Part model, mm, in its own coordinate system. Face numbers are marked on the shaded views. A direction names the side the tool comes from. Round coordinates to 2 decimals unless told otherwise and drop trailing zeros. Loops run counter-clockwise (first coordinate to the right, second up) from the corner with the lowest first, then second, coordinate; pieces in that order, holes last. Notation, with made-up numbers: (5, -26.5) - (27, -26.5) arc R23 ccw to (27, -1.5) - close; hole circle Ø1 at (30.25, -29). An arc over 180 degrees is marked (long way). Put each result on its own line as item: value.
from build123d import *

# Parameters (mm, degrees)
ESQUISSE1_R                  = 100
ESQUISSE1_R_2                = 4.25
ESQUISSE1_R_3                = 8
BOSS_EXTRU_1_DEPTH           = 40
ESQUISSE3_R                  = 5
ENL_V_MAT_EXTRU_2_DEPTH      = 41
ESQUISSE5_R                  = 15
ENL_V_MAT_EXTRU_3_DEPTH      = 30
ESQUISSE6_R                  = 33
ENL_V_MAT_EXTRU_4_DEPTH      = 5
ESQUISSE8_R                  = 17
ENL_V_MAT_EXTRU_5_DEPTH      = 20
R_P_TITION_CIRCULAIRE1_COUNT = 3


with BuildPart() as part:
    # Esquisse1 → Boss.-Extru.1 (new body)
    with BuildSketch(Plane(origin=(0, 0, 0), x_dir=(1, 0, 0), z_dir=(0, 1, 0))):
        with Locations(Location((0, 0, 0), (0, 0, 270))):  # turned: the seam where the file's is
            Circle(ESQUISSE1_R)
        with Locations(Location((-40.311740852, 7.648092634, 0), (0, 0, 270))):  # turned: the seam where the file's is
            Circle(ESQUISSE1_R_2, mode=Mode.SUBTRACT)
        with Locations(Location((-68.947262615, 13.080929779, 0), (0, 0, 270))):  # turned: the seam where the file's is
            Circle(ESQUISSE1_R_3, mode=Mode.SUBTRACT)
        with Locations(Location((45.802048801, 53.169616056, 0), (0, 0, 270))):  # turned: the seam where the file's is
            Circle(ESQUISSE1_R_3, mode=Mode.SUBTRACT)
        with Locations(Location((23.145213813, -66.250545836, 0), (0, 0, 270))):  # turned: the seam where the file's is
            Circle(ESQUISSE1_R_3, mode=Mode.SUBTRACT)
    extrude(amount=-BOSS_EXTRU_1_DEPTH)

    # Esquisse3 → Enlèv. mat.-Extru.2 (cut, through all)
    with BuildSketch(Plane(origin=(0, 0, 0), x_dir=(1, 0, 0), z_dir=(0, 1, 0))):
        with Locations(Location((0, 0, 0), (0, 0, 270))):  # turned: the seam where the file's is
            Circle(ESQUISSE3_R)
    extrude(amount=-ENL_V_MAT_EXTRU_2_DEPTH, mode=Mode.SUBTRACT)

    # Esquisse5 → Enlèv. mat.-Extru.3 (cut)
    with BuildSketch(Plane(origin=(0, 0, 0), x_dir=(1, 0, 0), z_dir=(0, 1, 0))):
        with Locations(Location((0, 0, 0), (0, 0, 270))):  # turned: the seam where the file's is
            Circle(ESQUISSE5_R)
    extrude(amount=-ENL_V_MAT_EXTRU_3_DEPTH, mode=Mode.SUBTRACT)

    # Esquisse6 → Enlèv. mat.-Extru.4 (cut)
    with BuildSketch(Plane(origin=(0, 0, 0), x_dir=(1, 0, 0), z_dir=(0, 1, 0))):
        with Locations(Location((0, 0, 0), (0, 0, 270))):  # turned: the seam where the file's is
            Circle(ESQUISSE6_R)
    extrude(amount=-ENL_V_MAT_EXTRU_4_DEPTH, mode=Mode.SUBTRACT)

    # Esquisse8 → Enlèv. mat.-Extru.5 (cut)
    with BuildSketch(Plane(origin=(0, 0, 0), x_dir=(1, 0, 0), z_dir=(0, 1, 0))):
        with Locations(Location((-68.773193764, 13.047904793, 0), (0, 0, 270))):  # turned: the seam where the file's is
            Circle(ESQUISSE8_R)
    enl_v_mat_extru_5 = extrude(amount=-ENL_V_MAT_EXTRU_5_DEPTH, mode=Mode.SUBTRACT)

    # Répétition circulaire1: Enlèv. mat.-Extru.5 ×3 about axis
    r_p_tition_circulaire1_axis = Axis((0, 0, 0), (0, 1, 0))
    for i in range(1, R_P_TITION_CIRCULAIRE1_COUNT):
        add(enl_v_mat_extru_5.rotate(r_p_tition_circulaire1_axis, i * 360 / R_P_TITION_CIRCULAIRE1_COUNT), mode=Mode.SUBTRACT)


solid = part.part
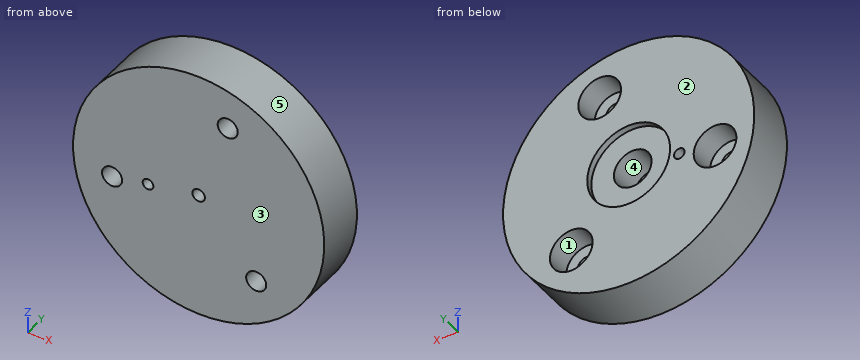
1. Band-saw the part on B-B (z = 67.5). List the corners of the cut face in (x, y).
A:
outline: (-73.78, -40) - (15.24, -40) - (15.24, -20) - (6.15, -20) - (6.15, 0) - (-73.78, 0) - close; (31.05, -40) - (73.78, -40) - (73.78, 0) - (40.03, 0) - (40.03, -20) - (31.05, -20) - close
2. Tool access for the marked faces 1 and 2: list every direction of +Z, -Z, +X, -X, +Y, -Y with a clear straight run to the whole face (end or side of a thin tool).
A:
face 1: +Y
face 2: +Z, -Z, +X, -X, +Y
3. Two-plate mould, pull along X, no slides. Class the marked faces 3, 4 and 5: pulls with the +X half, pulls with the -X half, needs draft (parallel to the pull), parting line crosses it, or undercut.
A:
face 3: needs draft
face 4: undercut
face 5: parting line crosses it
4. Pin check, flat tips, straight feed: P1, Ø10, axis at x = -7, y = -32, coming from the +Z side; P2, Ø10, axis at y = -32.5, z = -35.5, coming from the +X side; P3, Ø5, axis at y = -18, z = 58.5, coming from the -X side. Stop position of each tip, or through.
A:
P1: stops at z = 99.98
P2: stops at x = 95.24
P3: stops at x = -82.85
5. Probe line 1 along X through (y, z) = (-33, -10); line 2 along X through (y, z) = (-16.5, 0); line 3 along Y through (x, z) = (-28, 0.5). List the from-to ranges inside material, lowest first. Write a range as [from, to].
A:
line 1: x = [-99.5, -76.33], [-61.56, -43.85], [-36.77, 99.5]
line 2: x = [-100, -79.67], [-57.88, -15], [15, 100]
line 3: y = [-40, -5]
6. Band-saw the part on A-A (x = 0). List the corners of the cut face in (y, z).
A:
outline: (-40, -100) - (0, -100) - (0, -33) - (-5, -33) - (-5, -15) - (-30, -15) - (-30, -5) - (-40, -5) - close; (-40, 5) - (-30, 5) - (-30, 15) - (-5, 15) - (-5, 33) - (0, 33) - (0, 100) - (-40, 100) - close
7. Band-saw the part on D-D (x = -73). List the corners of the cut face in (y, z).
A:
outline: (-40, -68.34) - (0, -68.34) - (0, -29.51) - (-20, -29.51) - (-20, -19.98) - (-40, -19.98) - close; (-40, -6.18) - (-20, -6.18) - (-20, 3.42) - (0, 3.42) - (0, 68.34) - (-40, 68.34) - close
8. Band-saw the part on C-C (y = -12.5). List the corners of the cut face in (x, z).
A:
outline: circle Ø200 at (0, 0); hole circle Ø34 at (-68.77, -13.05); hole circle Ø8.5 at (-40.31, -7.65); hole circle Ø30 at (0, 0); hole circle Ø34 at (23.09, 66.08); hole circle Ø34 at (45.69, -53.04)
